from build123d import *

# Parameters (mm, degrees)
SKETCH1_R           = 3.6
SKETCH1_R_2         = 2.55
BOSS_EXTRUDE1_DEPTH = 3


with BuildPart() as part:
    # Sketch1 → Boss-Extrude1 (new body)
    with BuildSketch(Plane(origin=(0, 0, 0), x_dir=(1, 0, 0), z_dir=(0, 1, 0))):
        with BuildLine():
            Line((-29.75, 32.75), (29.75, 32.75))
            ThreePointArc((29.75, 32.75), (31.871320344, 31.871320344), (32.75, 29.75))
            Line((32.75, 29.75), (32.75, -29.75))
            ThreePointArc((32.75, -29.75), (31.871320344, -31.871320344), (29.75, -32.75))
            Line((29.75, -32.75), (-29.75, -32.75))
            ThreePointArc((-29.75, -32.75), (-31.871320344, -31.871320344), (-32.75, -29.75))
            Line((-32.75, -29.75), (-32.75, 29.75))
            ThreePointArc((-32.75, 29.75), (-31.871320344, 31.871320344), (-29.75, 32.75))
        make_face()
        with Locations(Location((-20, 19.85, 0), (0, 0, 270))):
            Circle(SKETCH1_R, mode=Mode.SUBTRACT)
        with Locations(Location((-19.85, 0, 0), (0, 0, 270))):
            Circle(SKETCH1_R, mode=Mode.SUBTRACT)
        with Locations(Location((-19.85, -20, 0), (0, 0, 270))):
            Circle(SKETCH1_R, mode=Mode.SUBTRACT)
        with Locations(Location((-19.85, 10, 0), (0, 0, 270))):
            Circle(SKETCH1_R_2, mode=Mode.SUBTRACT)
        with Locations(Location((-19.85, -10, 0), (0, 0, 90))):
            Circle(SKETCH1_R_2, mode=Mode.SUBTRACT)
        with Locations(Location((19.85, -20, 0), (0, 0, 90))):
            Circle(SKETCH1_R, mode=Mode.SUBTRACT)
        with Locations(Location((20, 19.85, 0), (0, 0, 90))):
            Circle(SKETCH1_R, mode=Mode.SUBTRACT)
        with Locations(Location((19.85, 10, 0), (0, 0, 90))):
            Circle(SKETCH1_R_2, mode=Mode.SUBTRACT)
        with Locations(Location((19.85, -10, 0), (0, 0, 270))):
            Circle(SKETCH1_R_2, mode=Mode.SUBTRACT)
        with Locations(Location((19.85, 0, 0), (0, 0, 270))):
            Circle(SKETCH1_R_2, mode=Mode.SUBTRACT)
        with Locations(Location((0, 0, 0), (0, 0, 270))):
            Circle(SKETCH1_R_2, mode=Mode.SUBTRACT)
        with Locations(Location((10, 0, 0), (0, 0, 270))):
            Circle(SKETCH1_R_2, mode=Mode.SUBTRACT)
        with Locations(Location((0, 10, 0), (0, 0, 90))):
            Circle(SKETCH1_R_2, mode=Mode.SUBTRACT)
        with Locations(Location((-10, 0, 0), (0, 0, 270))):
            Circle(SKETCH1_R_2, mode=Mode.SUBTRACT)
        with Locations(Location((0, -10, 0), (0, 0, 90))):
            Circle(SKETCH1_R_2, mode=Mode.SUBTRACT)
        with BuildLine():
            Line((-3.25, 29.2), (3.25, 29.2))
            ThreePointArc((3.25, 29.2), (4.75, 27.7), (3.25, 26.2))
            Line((3.25, 26.2), (-3.25, 26.2))
            ThreePointArc((-3.25, 26.2), (-4.75, 27.7), (-3.25, 29.2))
        make_face(mode=Mode.SUBTRACT)
        with BuildLine():
            Line((16.6, 29.2), (23.1, 29.2))
            ThreePointArc((23.1, 29.2), (24.6, 27.7), (23.1, 26.2))
            Line((23.1, 26.2), (16.6, 26.2))
            ThreePointArc((16.6, 26.2), (15.1, 27.7), (16.6, 29.2))
        make_face(mode=Mode.SUBTRACT)
        with BuildLine():
            Line((-16.6, 26.2), (-23.1, 26.2))
            ThreePointArc((-23.1, 26.2), (-24.6, 27.7), (-23.1, 29.2))
            Line((-23.1, 29.2), (-16.6, 29.2))
            ThreePointArc((-16.6, 29.2), (-15.1, 27.7), (-16.6, 26.2))
        make_face(mode=Mode.SUBTRACT)
        with BuildLine():
            Line((-16.6, -29.2), (-23.1, -29.2))
            ThreePointArc((-23.1, -29.2), (-24.6, -27.7), (-23.1, -26.2))
            Line((-23.1, -26.2), (-16.6, -26.2))
            ThreePointArc((-16.6, -26.2), (-15.1, -27.7), (-16.6, -29.2))
        make_face(mode=Mode.SUBTRACT)
        with BuildLine():
            Line((16.6, -26.2), (23.1, -26.2))
            ThreePointArc((23.1, -26.2), (24.6, -27.7), (23.1, -29.2))
            Line((23.1, -29.2), (16.6, -29.2))
            ThreePointArc((16.6, -29.2), (15.1, -27.7), (16.6, -26.2))
        make_face(mode=Mode.SUBTRACT)
        with BuildLine():
            Line((-3.25, -26.2), (3.25, -26.2))
            ThreePointArc((3.25, -26.2), (4.75, -27.7), (3.25, -29.2))
            Line((3.25, -29.2), (-3.25, -29.2))
            ThreePointArc((-3.25, -29.2), (-4.75, -27.7), (-3.25, -26.2))
        make_face(mode=Mode.SUBTRACT)
        with BuildLine():
            Line((-10, -17.35), (10, -17.35))
            ThreePointArc((10, -17.35), (12.5, -19.85), (10, -22.35))
            Line((10, -22.35), (-10, -22.35))
            ThreePointArc((-10, -22.35), (-12.5, -19.85), (-10, -17.35))
        make_face(mode=Mode.SUBTRACT)
        with BuildLine():
            Line((-10, 22.35), (10, 22.35))
            ThreePointArc((10, 22.35), (12.5, 19.85), (10, 17.35))
            Line((10, 17.35), (-10, 17.35))
            ThreePointArc((-10, 17.35), (-12.5, 19.85), (-10, 22.35))
        make_face(mode=Mode.SUBTRACT)
    extrude(amount=BOSS_EXTRUDE1_DEPTH)


solid = part.part
Here's how the part is built. I have some questions about the finished solid (model axes, mm). A direction names the side the tool comes from. Coordinates: 2 decimals unless noted, no trailing zeros. Order: outer loops, then holes, each group sorted by start corner. A loop starts at its lowest first (then second) coordinate and runs counter-clockwise, first axis right, second up.
Item 1: If we section it at A-A on z = 10: List the corners of the cut face in (x, y) for me, plus the area to 3 significant figures.
Result sheet:
outline: (-32.75, 0) - (-22.4, 0) - (-22.4, 3) - (-32.75, 3) - close; (-17.3, 0) - (-2.55, 0) - (-2.55, 3) - (-17.3, 3) - close; (2.55, 0) - (17.3, 0) - (17.3, 3) - (2.55, 3) - close; (22.4, 0) - (32.75, 0) - (32.75, 3) - (22.4, 3) - close
area: 151 mm2
Item 2: For P1, Ø8.5, axis at x = 20, z = -19.85, coming from the -Y side; P2, Ø3, axis at x = -19.85, z = -10, coming from the +Y side, each with a flat end and sliding along its axis, tell me the tip position at first contact or that it passes through.
Result sheet:
P1: stops at y = 0
P2: passes through
Item 3: If we mould it in two halves opening along Z, with no side actions, what happens to faces 1 (the face through (20, 1, 26.2)), 2 (the face through (31.85, 1.48, -31.89)), 3 (the face through (-31.85, 1.48, 31.89)), 4 (the face through (-32.75, 1, 0))? For each: +Z half, -Z half, draft (parallel to the pull), parting line (faces both ways), or undercut.
Result sheet:
face 1: undercut
face 2: -Z half
face 3: +Z half
face 4: draft
Item 4: If we section it at C-C on y = 1.5: State how many separate pieces and enclosed holes the cut face has, plus the area to 3 significant figures.
Result sheet:
separate pieces: 1
enclosed holes: 23
area: 3,480 mm2
Item 5: If we section it at B-B on z = -27.7: List the corners of the cut face in (x, y) for me.
Result sheet:
outline: (-32.75, 0) - (-24.6, 0) - (-24.6, 3) - (-32.75, 3) - close; (-15.1, 0) - (-4.75, 0) - (-4.75, 3) - (-15.1, 3) - close; (4.75, 0) - (15.1, 0) - (15.1, 3) - (4.75, 3) - close; (24.6, 0) - (32.75, 0) - (32.75, 3) - (24.6, 3) - close
Item 6: I need wall thicknesses on line 1 (X direction, y = 1.4, z = 20); line 2 (Z direction, x = 6.5, y = 0.6); line 3 (X direction, y = 1.8, z = 0). Which ranges of each line are inside material? Lowest first, please.
Result sheet:
line 1: x = -32.75 to -23.45, -16.25 to -12.5, 12.5 to 16.25, 23.45 to 32.75
line 2: z = -32.75 to -22.35, -17.35 to 17.35, 22.35 to 32.75
line 3: x = -32.75 to -23.45, -16.25 to -12.55, -7.45 to -2.55, 2.55 to 7.45, 12.55 to 17.3, 22.4 to 32.75
Item 7: For faces 5 (the face through (-7, 3, 0)), 6 (the face through (0, 1, -26.2)), which set-ups out of +Z, -Z, +X, -X, +Y, -Y let a thin tool reach every point of the face, with its end or its side?
Result sheet:
face 5: +Z, -Z, +X, -X, +Y
face 6: +Y, -Y
